Build history of the part. All positions in model axes, mm. Give positions to 0.01 mm unless a question says otherwise; leave off trailing zeros. Loops run counter-clockwise (first coordinate to the right, second up) from the corner with the lowest first, then second, coordinate; pieces in that order, holes last.
1) Flat gauge pins, fed straight in: P1, Ø21.5, axis at x = 14.351, y = 12.7, coming from the +Z side; P2, Ø1.5, axis at y = 18.5, z = 3, coming from the +X side; P3, Ø2, axis at y = 10.5, z = 2.5, coming from the +X side; P4, Ø4, axis at x = 88.9, y = 47.625, coming from the -Z side (3 decimals). Where does each tip first touch, or does it go through?
2) Band-saw the part on B-B on y = 9. List the corners of the cut face in (x, z).
3) Band-saw the part on A-A on x = 88.9. List the corners of the cut face in (y, z), then the cut area to 3 significant figures.
4) Band-saw the part on C-C on z = 2.6. State how many separate pieces and enclosed holes the cut face has, then the cut area to 3 significant figures.
5) Band-saw the part on D-D on x = 147. List the corners of the cut face in (y, z).
6) Wall check: line 1 (X direction, y = 12, z = 0.8); line 2 (X direction, y = 9, z = 2.35); line 3 (Y direction, x = 88.9, z = 2.35). Give the ranges that are in metal, low to high.
7) Two-plate mould, pull along X, no slides. Class faces 1 (the cylindrical face through (113.82, 55.83, 1.93)), 2 (the cylindrical face through (88.212, 44.526, 1.878)), 3 (the cylindrical face through (3.62, 3.82, 1.93)): +X half, -X half, draft (parallel to the pull), parting line (faces both ways), or undercut.
```python
from build123d import *

# Parameters (mm, degrees)
F0_W     = 177.8
F0_H     = 25.4
F0_R     = 6.6675
F0_R_2   = 3.175
F1_DEPTH = 3.81
F2_R     = 50.8
F3_R     = 12.7


with BuildPart() as f1:
    # F0 (on Top) → F1 (new body)
    with BuildSketch(Plane.XY):
        with Locations((88.9, 12.7)):
            Rectangle(F0_W, F0_H)
        with Locations((14.351, 12.7)):
            Circle(F0_R, mode=Mode.SUBTRACT)
        with Locations((163.449, 12.7)):
            Circle(F0_R, mode=Mode.SUBTRACT)
        Polygon((63.5, 57.15), (0, 25.4), (177.8, 25.4), (114.3, 57.15), align=None)
        with Locations((88.9, 47.625)):
            Circle(F0_R_2, mode=Mode.SUBTRACT)
    extrude(amount=F1_DEPTH)

    # F2
    f2_edges = [f1.edges().sort_by_distance(p)[0] for p in [
        (63.5, 57.15, 1.905),
        (114.3, 57.15, 1.905),
    ]]
    fillet(f2_edges, radius=F2_R)

    # F3
    f3_edges = [f1.edges().sort_by_distance(p)[0] for p in [
        (0, 25.4, 1.905),
        (0, 0, 1.905),
        (177.8, 0, 1.905),
        (177.8, 25.4, 1.905),
    ]]
    fillet(f3_edges, radius=F3_R)


solid = f1.part
```
Findings below:
1. P1: stops at z = 3.81
1. P2: stops at x = 177.8
1. P3: stops at x = 177.74
1. P4: passes through
2. outline: (0.55, 0) - (8.8, 0) - (8.8, 3.81) - (0.55, 3.81) - close; (19.9, 0) - (157.9, 0) - (157.9, 3.81) - (19.9, 3.81) - close; (169, 0) - (177.25, 0) - (177.25, 3.81) - (169, 3.81) - close
3. outline: (0, 0) - (44.45, 0) - (44.45, 3.81) - (0, 3.81) - close; (50.8, 0) - (57.15, 0) - (57.15, 3.81) - (50.8, 3.81) - close
3. area: 194 mm2
4. separate pieces: 1
4. enclosed holes: 3
4. area: 7,720 mm2
5. outline: (0, 0) - (40.8, 0) - (40.8, 3.81) - (0, 3.81) - close
6. line 1: x = 0.02 to 7.72, 20.98 to 156.82, 170.08 to 177.78
6. line 2: x = 0.55 to 8.8, 19.9 to 157.9, 169 to 177.25
6. line 3: y = 0 to 44.45, 50.8 to 57.15
7. face 1: +X half
7. face 2: undercut
7. face 3: -X half
